from build123d import *

# Parameters (mm, degrees)
CROQUIS1_R              = 3.5
SALIENTE_EXTRUIR1_DEPTH = 6
CROQUIS2_R              = 6
SALIENTE_EXTRUIR2_DEPTH = 3
CROQUIS3_R              = 2.5
CROQUIS3_R_2            = 1.5
CORTAR_EXTRUIR1_DEPTH   = 2
CROQUIS4_W              = 2
CROQUIS4_H              = 2
CORTAR_EXTRUIR2_DEPTH   = 4


with BuildPart() as part:
    # Croquis1 → Saliente-Extruir1 (new body)
    with BuildSketch(Plane.XY):
        with Locations((-4.754102012, 3.97833761)):
            Circle(CROQUIS1_R)
    extrude(amount=SALIENTE_EXTRUIR1_DEPTH)

    # Croquis2 → Saliente-Extruir2 (add)
    with BuildSketch(Plane(origin=(0, 0, 0), x_dir=(-1, 0, 0), z_dir=(0, 0, -1))):
        with Locations((4.754102012, 3.97833761)):
            Circle(CROQUIS2_R)
    extrude(amount=SALIENTE_EXTRUIR2_DEPTH)

    # Croquis3 → Cortar-Extruir1 (cut)
    with BuildSketch(Plane.XY.offset(6)):
        with Locations((-4.754102012, 3.97833761)):
            Circle(CROQUIS3_R)
        with Locations((-4.754102012, 3.97833761)):
            Circle(CROQUIS3_R_2, mode=Mode.SUBTRACT)
    extrude(amount=-CORTAR_EXTRUIR1_DEPTH, mode=Mode.SUBTRACT)

    # Croquis4 → Cortar-Extruir2 (cut, through all)
    with BuildSketch(Plane.XY):
        with Locations((-4.754102012, 8.97833761)):
            Rectangle(CROQUIS4_W, CROQUIS4_H)
        Polygon((-5.754102012, -0.02166239), (-3.754102012, -0.02166239), (-3.754102012, -2.02166239), (-4.754102012, -2.02166239), (-5.754102012, -2.02166239), align=None)
    extrude(amount=-CORTAR_EXTRUIR2_DEPTH, mode=Mode.SUBTRACT)


solid = part.part
Verification items for the finished model (mm, model axes). A direction names the side the tool comes from. Give positions to 0.01 mm unless a question says otherwise; leave off trailing zeros. Order: outer loops, then holes, each group sorted by start corner. A loop starts at its lowest first (then second) coordinate and runs counter-clockwise, first axis right, second up. Notation, with made-up numbers: M -12,-0.75 L -2,-0.75 A26 cw -2,36.25 Z; hole C 60.5,16.5 d11. An arc over 180 degrees is marked long. Use one line per item in the form item = value. Start each with the question number.
Q1. Section check D-D (x = -6.5). Enter the section's corners in (y, z), then the cut area to 3 significant figures.
Q2. Section check A-A (y = 8.25). Enter the section's corners in (x, z).
Q3. Access from +Z, -Z, +X, -X, +Y, -Y to the whole of each face (thin tool, end or side, straight path). Record for faces 4 (the flat face through (-5, 4, 6)), 5 (the cylindrical face through (-4.06, 2.65, 5.01)), 6 (the cylindrical face through (-10.753, 3.86, -1.479)), 7 (the flat face through (-5, -0.022, -1)), 8 (the flat face through (-5.754, 9, -1)).
Q4. Section check C-C (y = 3.5). Enter the section's corners in (x, z) (3 decimals).
Q5. Mould release check, pull along Y, two halves, no side actions. Record for faces 1 (the flat face through (-5, 7.978, -1)), 2 (the cylindrical face through (1.245, 4.096, -1.479)), 3 (the flat face through (-5, 2, 4)): +Y half, -Y half, draft (parallel to the pull), parting line (faces both ways), or undercut.
Q6. Go/stop test with flat-tipped pins: pin 1 Ø2 at (x, z) = (-8, -2) entering from +Y; pin 2 Ø1.5 at (x, y) = (-6, 5) entering from +Z; pin 3 Ø0.6 at (y, z) = (9, -1) entering from +X; pin 4 Ø1 at (y, z) = (7.5, 3.5) entering from +X. Record where each tip stops, or that it passes through.
Q7. Scan lines: line 1 along Z through (x, y) = (-8, 5.5); line 2 along Y through (x, z) = (-3.75, 5); line 3 along X through (y, z) = (8.5, -1). Record each from-to range of solid material in increasing order. Write a range as [from, to].
Q8. Section check B-B (z = -2.5). Enter the section's corners in (x, y).
Evaluation:
q1.outline = M -1.76,-3 L 9.72,-3 L 9.72,0 L 7.01,0 L 7.01,6 L 5.77,6 L 5.77,4 L 2.19,4 L 2.19,6 L 0.94,6 L 0.94,0 L -1.76,0 Z
q1.area = 63.7 mm2
q2.outline = M -8.97,-3 L -5.75,-3 L -5.75,0 L -8.97,0 Z; M -3.75,-3 L -0.54,-3 L -0.54,0 L -3.75,0 Z
q3.face_4 = +Z, +X, -X, +Y, -Y
q3.face_5 = +Z
q3.face_6 = +Z, -Z, -X
q3.face_7 = +Z, -Z, -Y
q3.face_8 = +Z, -Z, +Y
q4.outline = M -10.735,-3 L 1.227,-3 L 1.227,0 L -1.287,0 L -1.287,6 L -2.3,6 L -2.3,4 L -3.332,4 L -3.332,6 L -6.176,6 L -6.176,4 L -7.208,4 L -7.208,6 L -8.221,6 L -8.221,0 L -10.735,0 Z
q5.face_1 = +Y half
q5.face_2 = parting line
q5.face_3 = undercut
q6.pin_1 = 9.54
q6.pin_2 = 6
q6.pin_3 = -1.05
q6.pin_4 = -2.99
q7.line_1 = [-3, 0]
q7.line_2 = [0.63, 1.69], [2.86, 5.09], [6.27, 7.33]
q7.line_3 = [-8.7, -5.75], [-3.75, -0.81]
q8.outline = M -5.75,-1.94 L -5.75,-0.02 L -3.75,-0.02 L -3.75,-1.94 A6 ccw -3.75,9.89 L -3.75,7.98 L -5.75,7.98 L -5.75,9.89 A6 ccw Z
